Autodesk Inventor part; units mm, degrees
ref_plane "YZ Plane" through (0, 0, 0) normal (1, 0, 0) x (0, 1, 0)
ref_plane "XZ Plane" through (0, 0, 0) normal (0, 1, 0) x (-1, 0, 0)
ref_plane "XY Plane" through (0, 0, 0) normal (0, 0, 1) x (1, 0, 0)
sketch "Sketch1" plane through (0, 0, 0) normal (0, 1, 0) x (-1, 0, 0)
  line L0 (-254, -139.7) -> (254, -139.7)
  line L1 (254, -139.7) -> (254, 139.7)
  line L2 (254, 139.7) -> (-254, 139.7)
  line L3 (-254, 139.7) -> (-254, -139.7)
  line L4 (-254, -139.7) -> (254, 139.7) construction
  line L5 (254, -139.7) -> (-254, 139.7) construction
  point P0 (0, 0)
  dimension "d0" = 508
  dimension "d1" = 279.4
extrude "Extrusion1" add sketch "Sketch1" along normal blind 6.35
sketch "Sketch2" plane through (0, 6.35, 0) normal (0, 1, 0) x (1, 0, 0)
  line L0 (-254, 139.7) -> (-254, -139.7) construction
  line L1 (-254, -139.7) -> (254, -139.7) construction
  line L2 (254, -139.7) -> (254, 139.7) construction
  point P0 (0, 0)
  point P1 (-241.3, -127)
  point P2 (241.3, -127)
  point P3 (-241.3, -101.6)
  point P4 (241.3, -101.6)
  point P5 (-241.3, -76.2)
  point P6 (241.3, -76.2)
  point P7 (-241.3, -50.8)
  point P8 (241.3, -50.8)
  point P9 (-241.3, -25.4)
  point P10 (241.3, -25.4)
  point P11 (-241.3, 0)
  point P12 (241.3, 0)
  point P13 (-241.3, 25.4)
  point P14 (241.3, 25.4)
  point P15 (-241.3, 50.8)
  point P16 (241.3, 50.8)
  point P17 (-241.3, 76.2)
  point P18 (241.3, 76.2)
  point P19 (-241.3, 101.6)
  point P20 (241.3, 101.6)
  point P21 (-241.3, 127)
  point P22 (241.3, 127)
  dimension "d4" = 12.7
  dimension "d5" = 12.7
  dimension "d6" = 12.7
  dimension "d9" = 25.4
hole "Hole1" at (-241.3, 6.35, 127) at (241.3, 6.35, 127) at (-241.3, 6.35, 101.6) at (241.3, 6.35, 101.6) at (-241.3, 6.35, 76.2) at (241.3, 6.35, 76.2) at (-241.3, 6.35, 50.8) at (241.3, 6.35, 50.8) at (-241.3, 6.35, 25.4) at (-241.3, 6.35, 0) at (-241.3, 6.35, -25.4) at (-241.3, 6.35, -50.8) at (241.3, 6.35, -50.8) at (241.3, 6.35, -76.2) at (241.3, 6.35, -101.6) at (241.3, 6.35, -127) at (241.3, 6.35, 25.4) at (-241.3, 6.35, -76.2) direction (0, -1, 0) diameter 5.1054 end through all
sketch "Sketch3" plane through (0, 6.35, 0) normal (0, 1, 0) x (1, 0, 0)
  circle A0 centre (-241.3, 50.8) radius 2.5527 construction
  circle A1 centre (-241.3, 25.4) radius 2.5527 construction
  circle A2 centre (-241.3, 0) radius 2.5527 construction
  circle A3 centre (-241.3, -25.4) radius 2.5527 construction
  circle A4 centre (-241.3, -50.8) radius 2.5527 construction
  circle A5 centre (-241.3, -76.2) radius 2.5527 construction
  circle A6 centre (-241.3, -101.6) radius 2.5527 construction
  circle A7 centre (-241.3, -127) radius 2.5527 construction
  circle A8 centre (241.3, -127) radius 2.5527 construction
  circle A9 centre (241.3, -101.6) radius 2.5527 construction
  circle A10 centre (241.3, -76.2) radius 2.5527 construction
  circle A11 centre (241.3, -50.8) radius 2.5527 construction
  circle A12 centre (241.3, 50.8) radius 2.5527 construction
  circle A13 centre (241.3, 76.2) radius 2.5527 construction
  circle A14 centre (241.3, 101.6) radius 2.5527 construction
  circle A15 centre (241.3, 127) radius 2.5527 construction
  line L0 (-254, 139.7) -> (-254, -139.7) construction
  line L1 (-254, -139.7) -> (254, -139.7) construction
  line L2 (254, -139.7) -> (254, 139.7) construction
  line L3 (254, 139.7) -> (-254, 139.7) construction
  line L4 (-254, 139.7) -> (-254, -139.7) construction
  line L5 (254, 139.7) -> (-254, 139.7) construction
  line L6 (254, 139.7) -> (203.2, 139.7)
  line L7 (203.2, 139.7) -> (203.2, 114.3)
  line L8 (203.2, 114.3) -> (254, 114.3)
  line L9 (254, 114.3) -> (254, 139.7)
  line L10 (254, 139.7) -> (-254, 139.7) construction
  line L11 (-254, 139.7) -> (47.625, 139.7)
  line L12 (47.625, 139.7) -> (47.625, 101.6)
  line L13 (47.625, 101.6) -> (-254, 101.6)
  line L14 (-254, 101.6) -> (-254, 139.7)
  line L15 (47.625, 139.7) -> (85.725, 139.7)
  line L16 (85.725, 139.7) -> (85.725, 50.8)
  line L17 (85.725, 50.8) -> (47.625, 50.8)
  line L18 (47.625, 50.8) -> (47.625, 139.7)
  line L19 (254, -139.7) -> (254, 139.7) construction
  line L20 (254, 22.86) -> (228.6, 22.86)
  line L21 (228.6, 22.86) -> (228.6, -15.24)
  line L22 (228.6, -15.24) -> (254, -15.24)
  line L23 (254, -15.24) -> (254, 22.86)
  point P0 (0, 0)
  dimension "d30" = 25.4
  dimension "d31" = 50.8
  dimension "d42" = 206.375
  dimension "d43" = 38.1
  dimension "d44" = 88.9
  dimension "d45" = 168.275
  dimension "d46" = 25.4
  dimension "d47" = 38.1
  dimension "d48" = 124.46
extrude "Extrusion2" cut sketch "Sketch3" against normal through all
sketch "Sketch4" plane through (0, 6.35, 0) normal (0, 1, 0) x (1, 0, 0)
  line L0 (-224.6258, 34.925) -> (80.1742, 34.925) construction
  line L1 (80.1742, 34.925) -> (80.1742, -79.375) construction
  line L2 (80.1742, -79.375) -> (-224.6258, -79.375) construction
  line L3 (-224.6258, -79.375) -> (-224.6258, 34.925) construction
  circle A0 centre (203.2, -120.65) radius 14.2875
  circle A1 centre (105.0189, -107.95) radius 14.2875
  circle A2 centre (203.2, 76.2) radius 14.2875
  circle A3 centre (203.2, -120.65) radius 50.8 construction
  circle A4 centre (203.2, 76.2) radius 50.8 construction
  circle A5 centre (105.0189, -107.95) radius 31.75 construction
  circle A6 centre (203.2, -120.65) radius 41.275 construction
  circle A7 centre (203.2, 76.2) radius 41.275 construction
  line L4 (254, 22.86) -> (254, 114.3) construction
  line L5 (254, 114.3) -> (203.2, 114.3) construction
  line L6 (203.2, 114.3) -> (203.2, 139.7) construction
  line L7 (203.2, 139.7) -> (85.725, 139.7) construction
  line L8 (-254, 101.6) -> (-254, -139.7) construction
  line L9 (-254, -139.7) -> (254, -139.7) construction
  circle A8 centre (-241.3, -25.4) radius 2.5527 construction
  circle A9 centre (-241.3, -50.8) radius 2.5527 construction
  circle A10 centre (-241.3, -76.2) radius 2.5527 construction
  circle A11 centre (-241.3, -101.6) radius 2.5527 construction
  circle A12 centre (-241.3, -127) radius 2.5527 construction
  circle A13 centre (241.3, -127) radius 2.5527 construction
  circle A14 centre (241.3, -101.6) radius 2.5527 construction
  circle A15 centre (241.3, -76.2) radius 2.5527 construction
  circle A16 centre (241.3, -50.8) radius 2.5527 construction
  circle A17 centre (241.3, 50.8) radius 2.5527 construction
  circle A18 centre (241.3, 76.2) radius 2.5527 construction
  circle A19 centre (241.3, 101.6) radius 2.5527 construction
  circle A20 centre (105.0189, -107.95) radius 28.575 construction
  circle A21 centre (-241.3, 50.8) radius 2.5527
  line L10 (47.625, 50.8) -> (47.625, 101.6)
  line L11 (47.625, 101.6) -> (-254, 101.6)
  line L12 (85.725, 139.7) -> (85.725, 50.8)
  line L13 (85.725, 50.8) -> (47.625, 50.8)
  line L14 (254, -139.7) -> (254, -15.24)
  line L15 (254, -15.24) -> (228.6, -15.24)
  line L16 (228.6, -15.24) -> (228.6, 22.86)
  line L17 (228.6, 22.86) -> (254, 22.86)
  circle A22 centre (105.0189, 63.5) radius 14.2875
  circle A23 centre (105.0189, 63.5) radius 28.575 construction
  circle A24 centre (105.0189, 63.5) radius 31.75 construction
  circle A25 centre (6.2238, -101.6) radius 14.2875
  circle A26 centre (6.2238, 57.15) radius 14.2875
  circle A27 centre (6.2238, -101.6) radius 25.4 construction
  circle A28 centre (6.2238, -101.6) radius 22.225 construction
  circle A29 centre (6.2238, 57.15) radius 25.4 construction
  circle A30 centre (6.2238, 57.15) radius 22.225 construction
  point P0 (0, 0)
  point P1 (37.9738, 57.15)
  point P2 (37.9738, -101.6)
  point P3 (143.1189, -107.95)
  point P4 (143.1189, 63.5)
  dimension "d28" = 114.3
  dimension "d29" = 304.8
  dimension "d32" = 28.575
  dimension "d33" = 101.6
  dimension "d34" = 63.5
  dimension "d35" = 82.55
  dimension "d36" = 3.175
  dimension "d37" = 98.999
  dimension "d38" = 19.05
  dimension "d49" = 50.8
  dimension "d50" = 3.175
  dimension "d51" = 98.999
  dimension "d55" = 38.1
  dimension "d64" = 12.7
  dimension "d65" = 6.35
  dimension "d67" = 31.75
extrude "Extrusion3" cut sketch "Sketch4" against normal blind 25.4 contours A0 | A1 | A2 | A22 | A25 | A26
hole "Hole2" at (37.9738, 6.35, -57.15) at (37.9738, 6.35, 101.6) at (143.1189, 6.35, 107.95) at (143.1189, 6.35, -63.5) direction (0, -1, 0) diameter 5.1054 end through all
equation "\"d51\" = d37"
properties part number "GP3-001" material "Aluminum 6061"
Work out the finished part from the listing and answer in its coordinate system (mm). Round coordinates to 2 decimals unless told otherwise and drop trailing zeros. Write each loop counter-clockwise with the first axis right and the second up, starting at its lowest first coordinate (ties: lowest second). Pieces come first, ordered by that corner, then holes.
1) A cutting plane is placed at B-B on y = 1.25. Give the number of separate pieces and of enclosed holes in the cut face, and give its area (3 significant figures).
2) Determine the mould class of faces 1 (the face through (4, 0, 33)), 2 (the face through (210.88, 3.22, 108.6)) for opening direction Z: pulls with the +Z half, pulls with the -Z half, needs draft (parallel to the pull), parting line crosses it, or undercut.
3) Consider probe 1 along X at (y, z) = (1.5, 25.4); probe 2 along Z at (x, y) = (106, 1.75); probe 3 along Z at (x, y) = (99, 5.5). Determine where each line is inside the solid, lowest interval first.
4) Flat-ended cylindrical pins translate along their axes: P1, Ø4, axis at x = 62, z = -42, coming from the -Y side; P2, Ø1.5, axis at x = -78, y = 1.5, coming from the -Z side; P3, Ø3, axis at x = 236, y = 3, coming from the -Z side. Find the tip coordinate at first contact, or state that the pin passes through.
5) A cutting plane is placed at A-A on x = -64.5. Determine the outline of the cut face in (y, z), and give its area (3 significant figures).
Entries:
1. separate pieces: 1
1. enclosed holes: 27
1. area: 121,000 mm2
2. face 1: needs draft
2. face 2: undercut
3. probe 1: x = -254 to -243.85, -238.75 to 238.75, 243.85 to 254
3. probe 2: z = -139.7 to -77.75, -49.25 to 93.7, 122.2 to 139.7
3. probe 3: z = -139.7 to -76.46, -50.54 to 94.99, 120.91 to 139.7
4. P1: stops at y = 0
4. P2: stops at z = -101.6
4. P3: stops at z = -114.3
5. outline: (0, -101.6) - (6.35, -101.6) - (6.35, 139.7) - (0, 139.7) - close
5. area: 1,530 mm2
